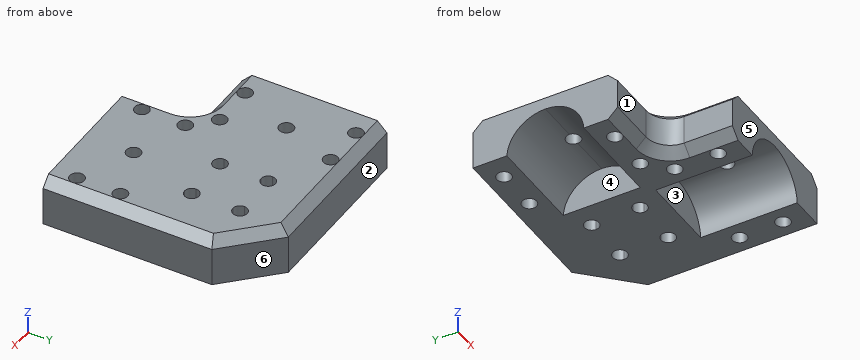
from build123d import *

# Parameters (mm, degrees)
BOSS_EXTRUDE1_DEPTH = 10
CUT_EXTRUDE1_DEPTH  = 20
CUT_EXTRUDE2_DEPTH  = 20
CUT_EXTRUDE3_DEPTH  = 20
SKETCH5_R           = 1.5
CUT_EXTRUDE4_DEPTH  = 20
FILLET1_R           = 5
CHAMFER1_SIZE       = 2
SKETCH6_R           = 1.5
CUT_EXTRUDE5_DEPTH  = 20


with BuildPart() as part:
    # Sketch1 → Boss-Extrude1 (new body)
    with BuildSketch(Plane.XY):
        Polygon((-30, -15), (-15, -15), (-15, -30), (15, -30), (15, 5), (5, 15), (-30, 15), align=None)
        with BuildLine():
            Line((-3.5, 5), (-6.5, 5))
            ThreePointArc((-6.5, 5), (-5, 6.5), (-3.5, 5))
        make_face(mode=Mode.SUBTRACT)
        with BuildLine():
            ThreePointArc((3.5, 5), (5, 6.5), (6.5, 5))
            Line((6.5, 5), (3.5, 5))
        make_face(mode=Mode.SUBTRACT)
    extrude(amount=BOSS_EXTRUDE1_DEPTH)

    # Sketch2 → Cut-Extrude1 (cut)
    with BuildSketch(Plane.XZ.offset(30)):
        with BuildLine():
            Line((0, 0), (7.984359711, 0))
            ThreePointArc((7.984359711, 0), (0, 7.5), (-7.984359711, 0))
            Line((-7.984359711, 0), (0, 0))
        make_face()
    extrude(amount=-CUT_EXTRUDE1_DEPTH, mode=Mode.SUBTRACT)

    # Sketch3 → Cut-Extrude2 (cut)
    with BuildSketch(Plane.ZY.offset(30)):
        with BuildLine():
            ThreePointArc((0, -7.984359711), (5.330951895, -5.477225575), (7.5, 0))
            ThreePointArc((7.5, 0), (5.330951895, 5.477225575), (0, 7.984359711))
            Line((0, 7.984359711), (0, 0))
            Line((0, 0), (0, -7.984359711))
        make_face()
    extrude(amount=-CUT_EXTRUDE2_DEPTH, mode=Mode.SUBTRACT)

    # Sketch4 → Cut-Extrude3 (cut)
    with BuildSketch(Plane(origin=(0, 0, 0), x_dir=(-1, 0, 0), z_dir=(0, 0, -1))):
        with BuildLine():
            ThreePointArc((3.5, 5), (5, 6.5), (6.5, 5))
            Line((6.5, 5), (3.5, 5))
        make_face()
        with BuildLine():
            Line((5, 5), (3.5, 5))
            ThreePointArc((3.5, 5), (3.939339828, 3.939339828), (5, 3.5))
            Line((5, 3.5), (5, 5))
        make_face()
        with BuildLine():
            Line((5, 5), (5, 3.5))
            ThreePointArc((5, 3.5), (6.060660172, 3.939339828), (6.5, 5))
            Line((6.5, 5), (5, 5))
        make_face()
        with BuildLine():
            Line((5, 5), (3.5, 5))
            ThreePointArc((3.5, 5), (3.939339828, 3.939339828), (5, 3.5))
            Line((5, 3.5), (5, 5))
        make_face()
        with BuildLine():
            Line((5, 5), (5, 3.5))
            ThreePointArc((5, 3.5), (6.060660172, 3.939339828), (6.5, 5))
            Line((6.5, 5), (5, 5))
        make_face()
        with BuildLine():
            ThreePointArc((5, -3.5), (3.939339828, -3.939339828), (3.5, -5))
            Line((3.5, -5), (5, -5))
            Line((5, -5), (5, -3.5))
        make_face()
        with BuildLine():
            Line((5, -5), (3.5, -5))
            ThreePointArc((3.5, -5), (5, -6.5), (6.5, -5))
            ThreePointArc((6.5, -5), (6.060660172, -3.939339828), (5, -3.5))
            Line((5, -3.5), (5, -5))
        make_face()
        with BuildLine():
            ThreePointArc((5, -3.5), (3.939339828, -3.939339828), (3.5, -5))
            Line((3.5, -5), (5, -5))
            Line((5, -5), (5, -3.5))
        make_face()
        with BuildLine():
            Line((5, -5), (3.5, -5))
            ThreePointArc((3.5, -5), (5, -6.5), (6.5, -5))
            ThreePointArc((6.5, -5), (6.060660172, -3.939339828), (5, -3.5))
            Line((5, -3.5), (5, -5))
        make_face()
        with BuildLine():
            Line((-5, 6.5), (-5, 5))
            Line((-5, 5), (-3.5, 5))
            ThreePointArc((-3.5, 5), (-3.939339828, 6.060660172), (-5, 6.5))
        make_face()
        with BuildLine():
            Line((-6.5, 5), (-5, 5))
            Line((-5, 5), (-5, 6.5))
            ThreePointArc((-5, 6.5), (-6.060660172, 6.060660172), (-6.5, 5))
        make_face()
        with BuildLine():
            Line((-5, 6.5), (-5, 5))
            Line((-5, 5), (-3.5, 5))
            ThreePointArc((-3.5, 5), (-3.939339828, 6.060660172), (-5, 6.5))
        make_face()
        with BuildLine():
            Line((-6.5, 5), (-5, 5))
            Line((-5, 5), (-5, 6.5))
            ThreePointArc((-5, 6.5), (-6.060660172, 6.060660172), (-6.5, 5))
        make_face()
        with BuildLine():
            ThreePointArc((-6.5, 5), (-6.060660172, 3.939339828), (-5, 3.5))
            Line((-5, 3.5), (-5, 5))
            Line((-5, 5), (-6.5, 5))
        make_face()
        with BuildLine():
            Line((-5, 5), (-5, 3.5))
            ThreePointArc((-5, 3.5), (-3.939339828, 3.939339828), (-3.5, 5))
            Line((-3.5, 5), (-5, 5))
        make_face()
        with BuildLine():
            ThreePointArc((-6.5, 5), (-6.060660172, 3.939339828), (-5, 3.5))
            Line((-5, 3.5), (-5, 5))
            Line((-5, 5), (-6.5, 5))
        make_face()
        with BuildLine():
            Line((-5, 5), (-5, 3.5))
            ThreePointArc((-5, 3.5), (-3.939339828, 3.939339828), (-3.5, 5))
            Line((-3.5, 5), (-5, 5))
        make_face()
        with BuildLine():
            Line((-5, -6.5), (-5, -5))
            Line((-5, -5), (-5, -3.5))
            ThreePointArc((-5, -3.5), (-6.5, -5), (-5, -6.5))
        make_face()
        with BuildLine():
            Line((-5, -3.5), (-5, -5))
            Line((-5, -5), (-3.5, -5))
            ThreePointArc((-3.5, -5), (-3.939339828, -3.939339828), (-5, -3.5))
        make_face()
        with BuildLine():
            Line((-3.5, -5), (-5, -5))
            Line((-5, -5), (-5, -6.5))
            ThreePointArc((-5, -6.5), (-3.939339828, -6.060660172), (-3.5, -5))
        make_face()
        with BuildLine():
            Line((-5, -3.5), (-5, -5))
            Line((-5, -5), (-3.5, -5))
            ThreePointArc((-3.5, -5), (-3.939339828, -3.939339828), (-5, -3.5))
        make_face()
        with BuildLine():
            Line((-3.5, -5), (-5, -5))
            Line((-5, -5), (-5, -6.5))
            ThreePointArc((-5, -6.5), (-3.939339828, -6.060660172), (-3.5, -5))
        make_face()
    extrude(amount=-CUT_EXTRUDE3_DEPTH, mode=Mode.SUBTRACT)

    # Sketch5 → Cut-Extrude4 (cut)
    with BuildSketch(Plane(origin=(0, 0, 0), x_dir=(-1, 0, 0), z_dir=(0, 0, -1))):
        with Locations((25, 11.492179856)):
            Circle(SKETCH5_R)
        with Locations((16, 11.492179856)):
            Circle(SKETCH5_R)
        with Locations((25, -11.492179856)):
            Circle(SKETCH5_R)
        with Locations((16, -11.492179856)):
            Circle(SKETCH5_R)
        with Locations((11.492179856, -16)):
            Circle(SKETCH5_R)
        with Locations((11.492179856, -25)):
            Circle(SKETCH5_R)
        with Locations(Location((-11.492179856, -16, 0), (0, 0, 180))):
            Circle(SKETCH5_R)
        with Locations((-11.492179856, -25)):
            Circle(SKETCH5_R)
    extrude(amount=-CUT_EXTRUDE4_DEPTH, mode=Mode.SUBTRACT)

    # Fillet1
    fillet1_edges = [part.edges().sort_by_distance(p)[0] for p in [
        (-15, -15, 5),
    ]]
    fillet(fillet1_edges, radius=FILLET1_R)

    # Chamfer1
    chamfer1_edges = [part.edges().sort_by_distance(p)[0] for p in [
        (-16.464466094, -16.464466094, 10),
        (-16.464466094, -16.464466094, 0),
        (-25, -15, 0),
        (15, -12.5, 10),
        (10, 10, 10),
        (-12.5, 15, 10),
        (-15, -25, 10),
        (-15, -25, 0),
        (-25, -15, 10),
    ]]
    chamfer(chamfer1_edges, length=CHAMFER1_SIZE)

    # Sketch6 → Cut-Extrude5 (cut)
    with BuildSketch(Plane.XY.offset(10)):
        with Locations((-20, 0)):
            Circle(SKETCH6_R)
        with Locations((0, -20)):
            Circle(SKETCH6_R)
    extrude(amount=-CUT_EXTRUDE5_DEPTH, mode=Mode.SUBTRACT)


solid = part.part
The listing builds one solid part. Answer for the finished solid, in the listing's coordinates (mm). Face numbers are marked on the shaded views. A direction names the side the tool comes from. Round coordinates to 2 decimals unless told otherwise and drop trailing zeros. Order: outer loops, then holes, each group sorted by start corner. A loop starts at its lowest first (then second) coordinate and runs counter-clockwise, first axis right, second up. Notation, with made-up numbers: (0.5, -7) -> (41.5, -7) arc R9 ccw to (41.5, 1) -> close; hole circle Ø8 at (5, 18.5). An arc over 180 degrees is marked (long way). Write each question's results on one line, items separated by ' | '. Start each with the question number.
Q1. Which of the six approach directions +Z, -Z, +X, -X, +Y, -Y give full straight-line access (tool end or side, diameter ignored) to the marked faces 1, 2 and 3?
Q2. The mould has two halves that part along Y. Classify the marked faces 4, 5 and 6: pulls with the +Y half, pulls with the -Y half, needs draft (parallel to the pull), parting line crosses it, or undercut.
Q3. Find section B-B (y = -16). Give the number of separate pieces and of enclosed holes in the cut face, then the cut area to 3 significant figures.
Q4. Straight lines are drawn through the part: probe 1 along X at (y, z) = (-12.5, 3); probe 2 along Y at (x, z) = (-22, 5.5); probe 3 along Y at (x, z) = (12, 6.5). For each, find the intervals that lie inside material, in ascending order. Write a range as from..to.
Q5. Find section A-A (x = 0). Determine the outline of the cut face in (y, z), then the cut area to 4 significant figures.
Q6. Find section D-D (x = 8.5). Determine the outline of the cut face in (y, z), then the cut area to 3 significant figures.
Q7. Each of these flat-tipped pins is pushed along its axis until it touches: pin 1 (2.5 mm diameter, centred on x = -25, y = -11.49, fed in from -Z); pin 2 (3.5 mm diameter, centred on x = 11.49, y = -16, fed in from +Z); pin 3 (5 mm diameter, centred on x = -24, z = 8, fed in from -Y); pin 4 (6 mm diameter, centred on y = 3.5, z = 2.5, fed in from -X). Where does it stop, or does it pass through?
Worked answers:
1) face 1: +Z, -Z, -X, -Y | face 2: +Z, -Z, +X, -X, +Y | face 3: -Z, -Y
2) face 4: undercut | face 5: pulls with the -Y half | face 6: pulls with the +Y half
3) separate pieces: 3 | enclosed holes: 0 | area: 160 mm2
4) probe 1: x = -30..-26.11, -23.89..-17.11, -14.89..-7.19, 7.19..15 | probe 2: y = -15..-5.29, 5.29..15 | probe 3: y = -30..-26.41, -23.59..-17.41, -14.59..8
5) outline: (-30, 7.5) -> (-21.5, 7.5) -> (-21.5, 10) -> (-30, 10) -> close; (-18.5, 7.5) -> (-10, 7.5) -> (-10, 0) -> (15, 0) -> (15, 8) -> (13, 10) -> (-18.5, 10) -> close | area: 290.5 mm2
6) outline: (-30, 0) -> (11.5, 0) -> (11.5, 8) -> (8.67, 10) -> (-30, 10) -> close | area: 412 mm2
7) pin 1: passes through | pin 2: stops at z = 10 | pin 3: stops at y = -15 | pin 4: stops at x = -10
